from build123d import *

# Parameters (mm, degrees)
SKETCH1_R           = 0.9
BOSS_EXTRUDE1_DEPTH = 7
FILLET1_R           = 2
FILLET2_R           = 1
FILLET3_R           = 0.5
SKETCH2_W           = 14.5
SKETCH2_H           = 14.5
CUT_EXTRUDE1_DEPTH  = 5.5
SKETCH3_R           = 7.8
BOSS_EXTRUDE2_DEPTH = 3.2
SKETCH5_R           = 0.75
CUT_EXTRUDE2_DEPTH  = 18.664653973
FILLET4_R           = 0.5
SKETCH6_R           = 5.8
CUT_EXTRUDE3_DEPTH  = 18.664653973


with BuildPart() as part:
    # Sketch1 → Boss-Extrude1 (new body)
    with BuildSketch(Plane.XY):
        Polygon((-8, 2), (-8, 8), (8, 8), (8, 2), (12, 2), (12, -2), (8, -2), (8, -8), (-8, -8), (-8, -2), (-12, -2), (-12, 2), align=None)
        with Locations((10, 0)):
            Circle(SKETCH1_R, mode=Mode.SUBTRACT)
        with Locations((-10, 0)):
            Circle(SKETCH1_R, mode=Mode.SUBTRACT)
    extrude(amount=BOSS_EXTRUDE1_DEPTH)

    # Fillet1
    fillet1_edges = [part.edges().sort_by_distance(p)[0] for p in [
        (-12, -2, 3.5),
        (-12, 2, 3.5),
        (12, -2, 3.5),
        (12, 2, 3.5),
    ]]
    fillet(fillet1_edges, radius=FILLET1_R - 0.0001)  # a hair under: the kernel refuses the full size

    # Fillet2
    fillet2_edges = [part.edges().sort_by_distance(p)[0] for p in [
        (8, -8, 3.5),
        (-8, -8, 3.5),
        (-8, 8, 3.5),
        (8, 8, 3.5),
    ]]
    fillet(fillet2_edges, radius=FILLET2_R)

    # Fillet3
    fillet3_edges = [part.edges().sort_by_distance(p)[0] for p in [
        (8, 2, 3.5),
        (8, -2, 3.5),
        (-8, -2, 3.5),
        (-8, 2, 3.5),
    ]]
    fillet(fillet3_edges, radius=FILLET3_R)

    # Sketch2 → Cut-Extrude1 (cut)
    with BuildSketch(Plane(origin=(0, 0, 0), x_dir=(-1, 0, 0), z_dir=(0, 0, -1))):
        Rectangle(SKETCH2_W, SKETCH2_H)
    extrude(amount=-CUT_EXTRUDE1_DEPTH, mode=Mode.SUBTRACT)

    # Sketch3 → Boss-Extrude2 (add)
    with BuildSketch(Plane.XY.offset(7)):
        with Locations(Location((0, 0, 0), (0, 0, 180))):
            Circle(SKETCH3_R)
    extrude(amount=BOSS_EXTRUDE2_DEPTH)

    # Sketch5 → Cut-Extrude2 (cut, through all)
    with BuildSketch(Plane(origin=(0, 0, 0), x_dir=(1, 0, 0), z_dir=(0, 1, 0))):
        with Locations(Location((0, -8.4, 0), (0, 0, 90))):
            Circle(SKETCH5_R)
    extrude(amount=CUT_EXTRUDE2_DEPTH, mode=Mode.SUBTRACT)

    # Fillet4
    fillet4_edges = [part.edges().sort_by_distance(p)[0] for p in [
        (7.8, 0, 10.2),
    ]]
    fillet(fillet4_edges, radius=FILLET4_R)

    # Sketch6 → Cut-Extrude3 (cut, through all)
    with BuildSketch(Plane.XY.offset(10.2)):
        Circle(SKETCH6_R)
    extrude(amount=-CUT_EXTRUDE3_DEPTH, mode=Mode.SUBTRACT)


solid = part.part
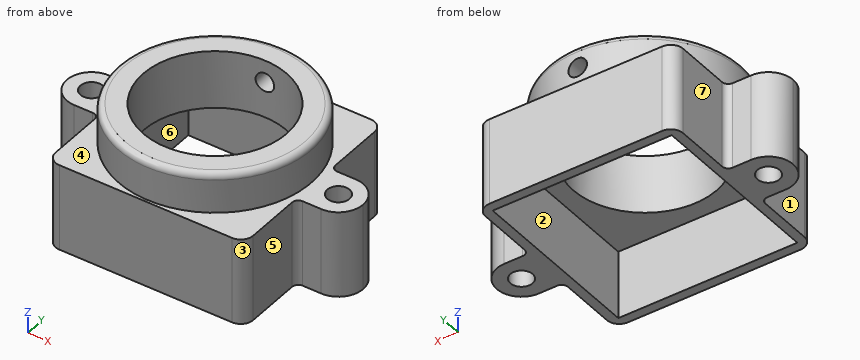
Read the model definition and answer for the solid it produces. Units are mm, in the model's axes. Face numbers are marked on the shaded views. A direction names the side the tool comes from. Give positions to 0.01 mm unless a question says otherwise; leave off trailing zeros. Write each loop counter-clockwise with the first axis right and the second up, starting at its lowest first coordinate (ties: lowest second). Pieces come first, ordered by that corner, then holes. Notation, with made-up numbers: (-11, -26) - (-7, -26) arc R11 ccw to (-7, -17) - close; hole circle Ø8 at (-2.75, 26.5). An arc over 180 degrees is marked (long way). Return JSON: item names as keys, results as strings.
Q1. A cutting plane is placed at B-B, the plane x = -10.5. Determine the outline of the cut face in (y, z), and give its area (3 significant figures).
Reply:
{"outline": "(-1.94, 0) - (-0.75, 0) - (-0.75, 7) - (-1.94, 7) - close; (0.75, 0) - (1.94, 0) - (1.94, 7) - (0.75, 7) - close", "area": "16.6 mm²"}
Q2. For the marked faces 4, 5, 6 and 7, determine the directions among +Z, -Z, +X, -X, +Y, -Y from which every point of the face is accessible in a straight line to the end or side of a thin tool.
Reply:
{"face 4": "+Z", "face 5": "+Z, -Z, +X, -Y", "face 6": "-Z", "face 7": "+Z, -Z, -X, +Y"}
Q3. For a pull along X with two mould halves and no side action, classify the marked faces 1, 2 and 3 as released by +X, released by -X, zero draft, split by the parting line, or undercut.
Reply:
{"face 1": "released by -X", "face 2": "undercut", "face 3": "released by +X"}
Q4. A cutting plane is placed at D-D, the plane z = 8.4. Determine the outline of the cut face in (x, y).
Reply:
{"outline": "(-0.75, 5.75) - (-0.75, 7.76) arc R7.8 ccw (long way) to (0.75, 7.76) - (0.75, 5.75) arc R5.8 cw (long way) to start"}
Q5. A cutting plane is placed at A-A, the plane z = 3.25. Count the separate pieces of the cut face and the enclosed holes in it, and give its area (3 significant figures).
Reply:
{"separate pieces": "1", "enclosed holes": "3", "area": "68.6 mm²"}
Q6. Consider line 1 along X through (y, z) = (-5.25, 5.25); line 2 along X through (y, z) = (0.25, 9.75); line 3 along X through (y, z) = (0.25, 3.75). Determine where each line is inside the solid, lowest interval first. Write a range as [from, to].
Reply:
{"line 1": "[-8, -7.25], [7.25, 8]", "line 2": "[-7.79, -5.79], [5.79, 7.79]", "line 3": "[-11.98, -10.86], [-9.14, -7.25], [7.25, 9.14], [10.86, 11.98]"}
Q7. Given P1, Ø1.4, axis at x = 0, z = 8.4, coming from the +Y side; P2, Ø1.7, axis at x = 9, z = 5, coming from the +Y side; P3, Ø2, axis at y = 1.5, z = 4, coming from the +X side, each flat-ended and moving along its own axis, determine where each tip first touches the part or whether it passes through.
Reply:
{"P1": "y = -5.76", "P2": "y = 2.14", "P3": "x = 11.94"}
